Source: CAD feature listing. Evaluate the final solid. Frame: model axes, mm. A direction names the side the tool comes from. Coordinates: 2 decimals unless noted, no trailing zeros. Loops run counter-clockwise (first coordinate to the right, second up) from the corner with the lowest first, then second, coordinate; pieces in that order, holes last.
```python
from build123d import *

# Parameters (mm, degrees)
BOSS_EXTRUDE1_DEPTH = 10
CUT_EXTRUDE1_DEPTH  = 7


with BuildPart() as part:
    # Sketch1 → Boss-Extrude1 (new body)
    with BuildSketch(Plane(origin=(0, 0, 0), x_dir=(1, 0, 0), z_dir=(0, 1, 0))):
        with BuildLine():
            Line((0.904649293, 0.632741314), (4.896029025, -5.073854375))
            Line((4.896029025, -5.073854375), (6, -5.073854375))
            Line((6, -5.073854375), (6, 9.926145625))
            Line((6, 9.926145625), (-6, 9.926145625))
            Line((-6, 9.926145625), (-6, -5.073854375))
            Line((-6, -5.073854375), (-4.896029025, -5.073854375))
            Line((-4.896029025, -5.073854375), (-0.904649293, 0.632741314))
            ThreePointArc((-0.904649293, 0.632741314), (0, 1.103970975), (0.904649293, 0.632741314))
        make_face()
    extrude(amount=BOSS_EXTRUDE1_DEPTH)

    # Sketch2 → Cut-Extrude1 (cut)
    with BuildSketch(Plane(origin=(0, 0, -9.926145625), x_dir=(-1, 0, 0), z_dir=(0, 0, -1))):
        with BuildLine():
            ThreePointArc((0, 7.1), (-2.1, 5), (0, 2.9))
            Line((0, 2.9), (0, 7.1))
        make_face()
        with BuildLine():
            Line((0, 7.1), (0, 2.9))
            ThreePointArc((0, 2.9), (1.48492424, 3.51507576), (2.1, 5))
            ThreePointArc((2.1, 5), (1.48492424, 6.48492424), (0, 7.1))
        make_face()
    extrude(amount=-CUT_EXTRUDE1_DEPTH, mode=Mode.SUBTRACT)


solid = part.part
```
Q1. Section query A-A on z = -3.75. Return the cut outline in (x, y), then the cut area to 3 significant figures.
Q2. Draft query along X for faces 1 (the flat face through (-6, 5, -3)), 2 (the flat face through (-2.93, 4.93, 2.26)), 3 (the flat face through (0, 0, -4)). Return one class per face: released by +X, released by -X, zero draft, split by the parting line, or undercut.
Q3. Material intervals for line 1 along Y through (x, z) = (-0.75, -7.5); line 2 along X through (y, z) = (4.5, 2.25); line 3 along X through (y, z) = (8.75, 4), sorted ascending.
Q4. Reachability of faces 4 (the flat face through (2.87, 4.93, 2.18)), 5 (the flat face through (0, 5, -2.926)), 6 (the flat face through (0, 10, -4)) from +Z, -Z, +X, -X, +Y, -Y: full face, straight path, thin tool, end or side. Return the list, or none.
Q5. Section query D-D on x = -4.5. Return the cut outline in (y, z).
Q6. Section query B-B on y = 2. Return the cut outline in (x, z), then the cut area to 3 significant figures.
Q7. Section query C-C on y = 3.25. Return the cut outline in (x, z), then the cut area to 3 significant figures.
Q8. First-contact query: pin 1 Ø2 at (x, y) = (0.5, 4.5) entering from -Z. Flat tip, straight axial feed; report the tip coordinate or a pass-through.
Resolved:
1. outline: (-6, 0) - (6, 0) - (6, 10) - (-6, 10) - close; hole circle Ø4.2 at (0, 5)
1. area: 106 mm2
2. face 1: released by -X
2. face 2: undercut
2. face 3: zero draft
3. line 1: y = 0 to 3.04, 6.96 to 10
3. line 2: x = -6 to -2.92, 2.92 to 6
3. line 3: x = -6 to -4.14, 4.14 to 6
4. face 4: +Z, +Y, -Y
4. face 5: -Z
4. face 6: +Z, -Z, +X, -X, +Y
5. outline: (0, -9.93) - (10, -9.93) - (10, 4.51) - (0, 4.51) - close
6. outline: (-6, -9.93) - (6, -9.93) - (6, 5.07) - (4.9, 5.07) - (0.9, -0.63) arc R1.1 cw to (-0.9, -0.63) - (-4.9, 5.07) - (-6, 5.07) - close
6. area: 146 mm2
7. outline: (-6, -9.93) - (-1.16, -9.93) - (-1.16, -2.93) - (1.16, -2.93) - (1.16, -9.93) - (6, -9.93) - (6, 5.07) - (4.9, 5.07) - (0.9, -0.63) arc R1.1 cw to (-0.9, -0.63) - (-4.9, 5.07) - (-6, 5.07) - close
7. area: 130 mm2
8. pin 1: stops at z = -2.93
